from build123d import *

# Parameters (mm, degrees)
BOSS_EXTRUDE1_DEPTH  = 7
M3_CLEARANCE_HOLE1_D = 3.2
CHAMFER2_SIZE        = 0.25
FILLET1_R            = 1


with BuildPart() as part:
    # Sketch1 → Boss-Extrude1 (new body)
    with BuildSketch(Plane(origin=(0, 0, 0), x_dir=(1, 0, 0), z_dir=(0, 1, 0))):
        with BuildLine():
            Line((0, 0), (-5, 0))
            Line((-5, 0), (-5, 9.065528002))
            Line((-5, 9.065528002), (-5, 27))
            ThreePointArc((-5, 27), (-3.828427125, 29.828427125), (-1, 31))
            Line((-1, 31), (0, 31))
            Line((0, 31), (0, 29))
            Line((0, 29), (-1, 29))
            ThreePointArc((-1, 29), (-3, 27), (-1, 25))
            Line((-1, 25), (0, 25))
            Line((0, 25), (0, 23))
            Line((0, 23), (-1, 23))
            ThreePointArc((-1, 23), (-3, 21), (-1, 19))
            Line((-1, 19), (0, 19))
            Line((0, 19), (0, 17))
            Line((0, 17), (-1, 17))
            ThreePointArc((-1, 17), (-3, 15), (-1, 13))
            Line((-1, 13), (0, 13))
            Line((0, 13), (0, 11))
            Line((0, 11), (-1, 11))
            ThreePointArc((-1, 11), (-3, 9), (-1, 7))
            Line((-1, 7), (0, 7))
            Line((0, 7), (0, 0))
        make_face()
    extrude(amount=BOSS_EXTRUDE1_DEPTH)

    # M3 Clearance Hole1 (through all)
    with Locations(Plane.ZY.offset(5)):
        with Locations((-3.5, 3.5)):
            Hole(M3_CLEARANCE_HOLE1_D / 2)

    # Chamfer2
    chamfer2_edges = [part.edges().sort_by_distance(p)[0] for p in [
        (-5, 3.5, -1.9),
        (0, 3.5, -1.9),
    ]]
    chamfer(chamfer2_edges, length=CHAMFER2_SIZE)

    # Fillet1
    fillet1_edges = [part.edges().sort_by_distance(p)[0] for p in [
        (-5, 3.5, 0),
    ]]
    fillet(fillet1_edges, radius=FILLET1_R)


solid = part.part
Geometry: final body of the model. Coordinates: model frame, mm. A direction names the side the tool comes from. Round coordinates to 2 decimals unless told otherwise and drop trailing zeros. Write each loop counter-clockwise with the first axis right and the second up, starting at its lowest first coordinate (ties: lowest second). Pieces come first, ordered by that corner, then holes. Notation, with made-up numbers: M 80,11.25 L 117,11.25 A22 cw 117,39.25 Z; hole C 19.5,74.5 d7. An arc over 180 degrees is marked long. Write item = value, one per line.
Item 1: Section query B-B on z = -3.5. Return loops of the section in (x, y), then the cut area to 3 significant figures.
Findings:
outline = M -5,0 L 0,0 L 0,1.65 L -0.25,1.9 L -4.75,1.9 L -5,1.65 Z; M -5,5.35 L -4.75,5.1 L -0.25,5.1 L 0,5.35 L 0,7 L -5,7 Z
area = 18.9 mm^2
Item 2: Access query for faces 1 (the face through (-5, 3, -14)), 2 (the face through (-0.5, 3.5, -13)). Directions: +Z, -Z, +X, -X, +Y, -Y. A direction counts if a zero-diameter tool reaches every point of the face in a straight line with its end or side. Return the directions, or none.
Findings:
face_1 = +Z, -Z, -X, +Y, -Y
face_2 = +X, +Y, -Y
Item 3: Section query D-D on y = 0.5. Return loops of the section in (x, z), then the cut area to 3 significant figures.
Findings:
outline = M -5,-27 A4 ccw -1,-31 L 0,-31 L 0,-29 L -1,-29 A2 cw -1,-25 L 0,-25 L 0,-23 L -1,-23 A2 cw -1,-19 L 0,-19 L 0,-17 L -1,-17 A2 cw -1,-13 L 0,-13 L 0,-11 L -1,-11 A2 cw -1,-7 L 0,-7 L 0,0 L -4,0 A1 ccw -5,-1 Z
area = 110 mm^2
Item 4: Material intervals for line 1 along Z through (x, y) = (-0.4, 1.25); line 2 along Z through (x, y) = (-1.4, 4.5); line 3 along Y through (x, z) = (-1.9, -3.5), sorted ascending. Write a range as [from, to].
Findings:
line_1 = [-31, -29], [-25, -23], [-19, -17], [-13, -11], [-7, 0]
line_2 = [-30.98, -28.96], [-25.04, -22.96], [-19.04, -16.96], [-13.04, -10.96], [-7.04, -4.75], [-2.25, 0]
line_3 = [0, 1.9], [5.1, 7]
Item 5: Section query C-C on x = -1.55. Return loops of the section in (y, z), then the cut area to 3 significant figures.
Findings:
outline = M 0,-30.96 L 7,-30.96 L 7,-28.92 L 0,-28.92 Z; M 0,-25.08 L 7,-25.08 L 7,-22.92 L 0,-22.92 Z; M 0,-19.08 L 7,-19.08 L 7,-16.92 L 0,-16.92 Z; M 0,-13.08 L 7,-13.08 L 7,-10.92 L 0,-10.92 Z; M 0,-7.08 L 7,-7.08 L 7,0 L 0,0 Z; hole C 3.5,-3.5 d3.2
area = 101 mm^2
Item 6: Pull-direction query (Y, two-part tool) for faces 3 (the face through (-2.47, 4.85, -4.36)), 4 (the face through (-3, 7, -16)), 5 (the face through (-3, 0, -16)), 6 (the face through (-3, 3, -15)); classes: pulls with the +Y half, pulls with the -Y half, needs draft (parallel to the pull), parting line crosses it, or undercut.
Findings:
face_3 = undercut
face_4 = pulls with the +Y half
face_5 = pulls with the -Y half
face_6 = needs draft
